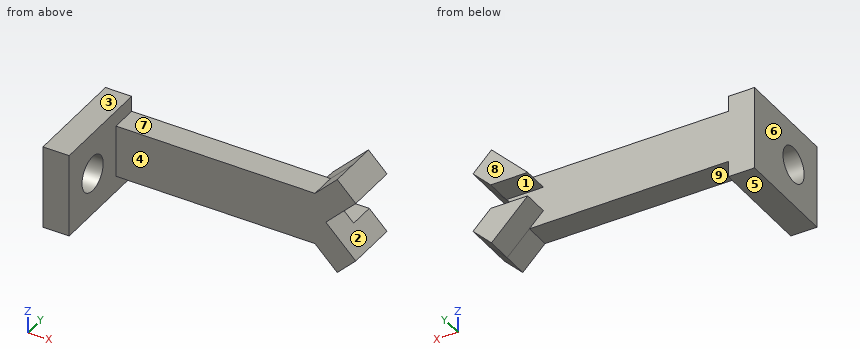
from build123d import *

# Parameters (mm, degrees)
BOSS_EXTRUDE1_DEPTH          = 3.175
BOSS_EXTRUDE2_DEPTH          = 3.175
SKETCH3_W                    = 3.175
SKETCH3_H                    = 10.16
BOSS_EXTRUDE3_DEPTH          = 12.7
F_18_0_1695_DIAMETER_HOLE1_D = 4.3053


with BuildPart() as part:
    # Sketch1 → Boss-Extrude1 (new body)
    with BuildSketch(Plane(origin=(0, 0, 0), x_dir=(1, 0, 0), z_dir=(0, 1, 0))):
        Polygon((20.825839478, -3.654842125), (17.191471303, -0.02047395), (-11.428656758, -0.02047395), (-11.428656758, -3.19547395), (15.876343242, -3.19547395), (18.580775448, -5.899906155), align=None)
    boss_extrude1 = extrude(amount=BOSS_EXTRUDE1_DEPTH)

    # Mirror1: Boss-Extrude1 across plane
    add(boss_extrude1.mirror(Plane(origin=(-11.428656758, 3.175, 0.02047395), x_dir=(1, 0, 0), z_dir=(0, 0, 1))))

    # Sketch2 → Boss-Extrude2 (add)
    with BuildSketch(Plane(origin=(0, 3.175, 0), x_dir=(1, 0, 0), z_dir=(0, 1, 0))):
        Polygon((18.580775448, -5.899906155), (14.18553725, -1.504667957), (18.675665311, -1.504667957), (20.825839478, -3.654842125), align=None)
        Polygon((18.675665311, 1.463720058), (20.825839478, 3.613894225), (18.580775448, 5.858958256), (14.18553725, 1.463720058), align=None)
    extrude(amount=BOSS_EXTRUDE2_DEPTH)

    # Sketch3 → Boss-Extrude3 (add)
    with BuildSketch(Plane(origin=(0, 3.175, 0), x_dir=(1, 0, 0), z_dir=(0, 1, 0))):
        with Locations((-9.841156758, 0)):
            Rectangle(SKETCH3_W, SKETCH3_H)
    extrude(amount=-BOSS_EXTRUDE3_DEPTH)

    # #18 (0.1695) Diameter Hole1 (through all)
    with Locations(Plane(origin=(-8.253656758, 0, 0), x_dir=(0, 0, -1), z_dir=(1, 0, 0))):
        with Locations((0, -4.7625)):
            Hole(F_18_0_1695_DIAMETER_HOLE1_D / 2)


solid = part.part
Work out the finished part from the listing and answer in its coordinate system (mm). Face numbers are marked on the shaded views. A direction names the side the tool comes from. Coordinates: 2 decimals unless noted, no trailing zeros. Order: outer loops, then holes, each group sorted by start corner. A loop starts at its lowest first (then second) coordinate and runs counter-clockwise, first axis right, second up. Notation, with made-up numbers: (6.25, 83) - (14.25, 83) arc R17 cw to (14.25, 99) - close; hole circle Ø7 at (0.5, 31). An arc over 180 degrees is marked (long way). Put each result on its own line as item: value. Start each with the question number.
1) For the marked faces 1, 2, 3, 4 and 5, determine the directions among +Z, -Z, +X, -X, +Y, -Y from which every point of the face is accessible in a straight line to the end or side of a thin tool.
2) Find the intervals of material crossed by line 1 (Y direction, x = -9.35, z = 0) (3 decimals); line 2 (Y direction, x = 7, z = 2) (3 decimals); line 3 (Y direction, x = 19.5, z = -2.5), in increasing order. Write a range as from..to.
3) For a pull along X with two mould halves and no side action, classify the marked faces 6, 7, 8 and 9 as released by +X, released by -X, zero draft, split by the parting line, or undercut.
4) Find section D-D (z = -2.75). Give the vertices of the cut face in (x, y) (3 decimals).
5) Flat-ended cylindrical pins translate along their axes: pin 1 (1 mm diameter, centred on x = 15.5, y = 4, fed in from +Z); pin 2 (3 mm diameter, centred on x = 5, y = 4, fed in from -Z); pin 3 (1.5 mm diameter, centred on x = -6.5, z = 3, fed in from -Y); pin 4 (3.5 mm diameter, centred on y = -4.76, z = 0, fed in from -X). Find the tip coordinate at first contact, or state that the pin passes through.
6) Find section A-A (y = 4.5). Give the vertices of the cut face in (x, z), plus the area to 3 significant figures.
7) Find section C-C (y = -3.75). Give the vertices of the cut face in (x, z), plus the area to 3 significant figures.
8) Find section B-B (z = -0.75). Give the vertices of the cut face in (x, y) (3 decimals), plus the area to 3 significant figures.
Results list:
1. face 1: +X, -X, +Y
1. face 2: +X, +Y, -Y
1. face 3: +Z, -X, +Y, -Y
1. face 4: +Z, -Z, +X, -Y
1. face 5: -Z, -X, +Y, -Y
2. line 1: y = -9.525..-6.915, -2.61..3.175
2. line 2: y = 0..3.175
2. line 3: y = 0..6.35
3. face 6: released by -X
3. face 7: undercut
3. face 8: zero draft
3. face 9: undercut
4. outline: (-11.429, -9.525) - (-8.254, -9.525) - (-8.254, 0) - (19.962, 0) - (19.962, 6.35) - (15.472, 6.35) - (15.472, 3.175) - (-11.429, 3.175) - close
5. pin 1: stops at z = 3.32
5. pin 2: stops at z = -3.15
5. pin 3: stops at y = 0
5. pin 4: passes through
6. outline: (14.19, -1.46) - (18.58, -5.86) - (20.83, -3.61) - (18.68, -1.46) - close; (14.19, 1.5) - (18.68, 1.5) - (20.83, 3.65) - (18.58, 5.9) - close
6. area: 29.4 mm^2
7. outline: (-11.43, -5.08) - (-8.25, -5.08) - (-8.25, -1.9) - (-11.43, -1.9) - close; (-11.43, 1.9) - (-8.25, 1.9) - (-8.25, 5.08) - (-11.43, 5.08) - close
7. area: 20.2 mm^2
8. outline: (-11.429, -9.525) - (-8.254, -9.525) - (-8.254, -6.78) - (-11.429, -6.78) - close; (-11.429, -2.745) - (-8.254, -2.745) - (-8.254, 0) - (17.962, 0) - (17.962, 3.175) - (-11.429, 3.175) - close
8. area: 111 mm^2
